```python
from build123d import *

# Parameters (mm, degrees)
F1_DEPTH = 35
F2_R     = 2


with BuildPart() as f1:
    # F0 (on Right) → F1 (new body)
    with BuildSketch(Plane.YZ):
        Polygon((-60, 4.5), (-60, 4), (-70, 4), (-70, 3.5), (-80, 3.5), (-80, 3), (-90, 3), (-90, 2.5), (-100, 2.5), (-100, 2), (-110, 2), (-110, 1.5), (-120, 1.5), (-120, 1), (-130, 1), (-130, 0), (0, 0), (0, 7), (-10, 7), (-10, 6.5), (-20, 6.5), (-20, 6), (-30, 6), (-30, 5.5), (-40, 5.5), (-40, 5), (-50, 5), (-50, 4.5), align=None)
    extrude(amount=F1_DEPTH)

    # F2
    f2_edges = [f1.edges().sort_by_distance(p)[0] for p in [
        (35, 0, 3.5),
        (35, -130, 0.5),
        (0, -130, 0.5),
        (0, 0, 3.5),
    ]]
    fillet(f2_edges, radius=F2_R)


solid = f1.part
```
For this review, take the finished solid that the model builds, in its own axes (mm). A direction names the side the tool comes from. Round coordinates to 2 decimals unless told otherwise and drop trailing zeros. Write each loop counter-clockwise with the first axis right and the second up, starting at its lowest first coordinate (ties: lowest second). Pieces come first, ordered by that corner, then holes. Notation, with made-up numbers: (52.5, 61) - (75.5, 61) arc R15 ccw to (75.5, 89) - close; hole circle Ø7 at (-20.75, -28.75). An arc over 180 degrees is marked (long way). Answer as a JSON object with one key per item and string values.
1. We need section B-B on y = -116.5. Give the boundary of the cut face in (x, z), then the cut area to 3 significant figures.
Response values:
{"outline": "(0, 0) - (35, 0) - (35, 1.5) - (0, 1.5) - close", "area": "52.5 mm2"}
2. To check wall thickness, follow line 1 along Z through (x, y) = (6, -34.5); line 2 along Z through (x, y) = (14, -97); line 3 along Y through (x, z) = (11, 2.25). State the ranges of each line that lie inside material, in increasing order.
Response values:
{"line 1": "z = 0 to 5.5", "line 2": "z = 0 to 2.5", "line 3": "y = -100 to 0"}
3. For pin 1 Ø1.5 at (x, y) = (4, -36) entering from +Z; pin 2 Ø5 at (x, y) = (21.5, -101.5) entering from -Z; pin 3 Ø5 at (x, y) = (24, -75) entering from +Z; pin 4 Ø8 at (x, y) = (26, -16.5) entering from +Z, all flat-tipped, find the tip position at first contact; note any pin that passes through.
Response values:
{"pin 1": "stops at z = 5.5", "pin 2": "stops at z = 0", "pin 3": "stops at z = 3.5", "pin 4": "stops at z = 6.5"}
4. Tool access review of faces 1 (the face through (0, -52, 3)), 2 (the face through (17, -35, 5.5)): name each direction out of +Z, -Z, +X, -X, +Y, -Y from which nothing blocks a thin tool from reaching the whole face with its end or side.
Response values:
{"face 1": "+Z, -Z, -X, +Y, -Y", "face 2": "+Z, +X, -X, -Y"}
5. We need section C-C on y = -97. Give the boundary of the cut face in (x, z).
Response values:
{"outline": "(0, 0) - (35, 0) - (35, 2.5) - (0, 2.5) - close"}
6. We need section A-A on x = 13.5. Give the boundary of the cut face in (y, z).
Response values:
{"outline": "(-130, 0) - (0, 0) - (0, 7) - (-10, 7) - (-10, 6.5) - (-20, 6.5) - (-20, 6) - (-30, 6) - (-30, 5.5) - (-40, 5.5) - (-40, 5) - (-50, 5) - (-50, 4.5) - (-60, 4.5) - (-60, 4) - (-70, 4) - (-70, 3.5) - (-80, 3.5) - (-80, 3) - (-90, 3) - (-90, 2.5) - (-100, 2.5) - (-100, 2) - (-110, 2) - (-110, 1.5) - (-120, 1.5) - (-120, 1) - (-130, 1) - close"}
